Model file for the job. Use its own axes, mm. Face numbers are marked on the shaded views. A direction names the side the tool comes from. Round coordinates to 2 decimals unless told otherwise and drop trailing zeros. Order: outer loops, then holes, each group sorted by start corner. A loop starts at its lowest first (then second) coordinate and runs counter-clockwise, first axis right, second up. Notation, with made-up numbers: (85, 37) - (101, 37) arc R19 ccw to (101, 62) - close; hole circle Ø6 at (-17.5, 5.5). An arc over 180 degrees is marked (long way). Put each result on its own line as item: value. Start each with the question number.
Item 1: Probe probe 1 along Z at (x, y) = (2.5, -1.4); probe 2 along Y at (x, z) = (3.5, -4.5); probe 3 along Y at (x, z) = (6, -2.75). List the from-to ranges inside material, lowest first.
Item 2: Saw through at A-A on z = -4. List the corners of the cut face in (x, y).
Item 3: Saw through at D-D on z = -6. List the corners of the cut face in (x, y), plus the area to 3 significant figures.
Item 4: Which spindle directions (+Z, -Z, +X, -X, +Y, -Y) get a long thin tool onto all of the face, cutting with end or side? Do the marked faces 4, 5 and 6. Say none if no direction does.
Item 5: Pin check, flat tips, straight feed: pin 1 Ø3 at (x, z) = (3.5, -4.5) entering from -Y; pin 2 Ø1.5 at (y, z) = (2, -2) entering from +X; pin 3 Ø1 at (x, y) = (3, -1.5) entering from +Z. Stop position of each tip, or through.
Item 6: Mould opens along Z. For the marked faces 1, 2 and 3 say: pulls with the +Z half, pulls with the -Z half, needs draft (parallel to the pull), parting line crosses it, or undercut.
Item 7: Saw through at C-C on x = 5.25. List the corners of the cut face in (y, z), plus the area to 3 significant figures.
Item 8: Saw through at B-B on y = 1. List the corners of the cut face in (x, z).
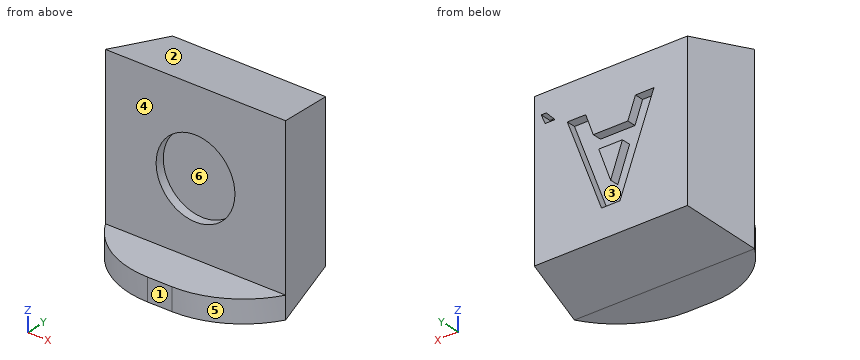
```python
from build123d import *

# Parameters (mm, degrees)
SKETCH1_W               = 8
SKETCH1_H               = 8
BOSS_EXTRUDE1_DEPTH     = 3
CUT_EXTRUDE1_DEPTH      = 12.704699911
CUT_EXTRUDE1_DEPTH_BACK = 12.704699911
CUT_EXTRUDE2_DEPTH      = 11
SKETCH4_R               = 1.75
CUT_EXTRUDE3_DEPTH      = 0.4
SKETCH5_W               = 8
SKETCH5_H               = 1
BOSS_EXTRUDE2_DEPTH     = 2
FILLET1_R               = 4
CUT_EXTRUDE4_DEPTH      = 0.4
CUT_EXTRUDE5_DEPTH      = 0.5


with BuildPart() as part:
    # Sketch1 → Boss-Extrude1 (new body)
    with BuildSketch(Plane(origin=(0, 0, 0), x_dir=(1, 0, 0), z_dir=(0, 1, 0))):
        with Locations((4, 4)):
            Rectangle(SKETCH1_W, SKETCH1_H)
    extrude(amount=BOSS_EXTRUDE1_DEPTH)

    # Sketch2 → Cut-Extrude1 (cut, two sides: drawn at the far end of the back side and taken through both)
    with BuildSketch(Plane.XY.offset(-CUT_EXTRUDE1_DEPTH_BACK)):
        Polygon((0, 0), (0.6, 3), (0, 3), align=None)
        Polygon((8, 0), (7.4, 3), (8, 3), align=None)
    extrude(amount=CUT_EXTRUDE1_DEPTH + CUT_EXTRUDE1_DEPTH_BACK, mode=Mode.SUBTRACT)

    # Sketch3 → Cut-Extrude2 (cut)
    with BuildSketch(Plane(origin=(0, 0, 0), x_dir=(0, 0, -1), z_dir=(1, 0, 0))):
        Polygon((0, 0), (0.6, 3), (0, 3), align=None)
        Polygon((8, 3), (7.4, 3), (8, 0), align=None)
    extrude(amount=CUT_EXTRUDE2_DEPTH, mode=Mode.SUBTRACT)

    # Sketch4 → Cut-Extrude3 (cut)
    with BuildSketch(Plane.XZ):
        with Locations(Location((4, -3.75, 0), (0, 0, 270))):
            Circle(SKETCH4_R)
    extrude(amount=-CUT_EXTRUDE3_DEPTH, mode=Mode.SUBTRACT)

    # Sketch5 → Boss-Extrude2 (add)
    with BuildSketch(Plane.XZ):
        with Locations((4, -7.5)):
            Rectangle(SKETCH5_W, SKETCH5_H)
    extrude(amount=BOSS_EXTRUDE2_DEPTH)

    # Fillet1
    # the kernel refuses this fillet: 4 mm, written as the material it takes off along each edge
    with BuildSketch(Plane(origin=(8, -2, -16.660254038), x_dir=(0, 1, 0), z_dir=(0, 0, 1)), Plane(origin=(0, -2, 1.660254038), x_dir=(0, 1, 0), z_dir=(0, 0, -1))) as fillet1_piece_1:
        with BuildLine():
            CenterArc((4, 3.464101615), FILLET1_R, 180, 60)
            Line((0, 3.464101615), (-0.08, 3.464101615))
            Line((-0.08, 3.464101615), (-0.08, 0))
            Line((-0.08, 0), (0, -0.08))
            ThreePointArc((0, -0.08), (1, -0.08), (1.96, -0.069282032))
            Line((1.96, -0.069282032), (2, 0))
        make_face()
    extrude(amount=18.320508076, mode=Mode.SUBTRACT)

    # Sketch6 → Cut-Extrude4 (cut)
    with BuildSketch(Plane(origin=(0, 3, 0), x_dir=(1, 0, 0), z_dir=(0, 1, 0))):
        Polygon((5.933857302, 2.141652068), (5.118152174, 2.141652068), (4.780812431, 3.064728992), (3.24555602, 3.064728992), (2.908216277, 2.141652068), (2.087703456, 2.141652068), (3.599722687, 6.141652068), (4.414626533, 6.141652068), align=None)
        Polygon((4.536421405, 3.731395658), (4.010780379, 5.167293094), (3.486741918, 3.731395658), align=None, mode=Mode.SUBTRACT)
    extrude(amount=-CUT_EXTRUDE4_DEPTH, mode=Mode.SUBTRACT)

    # Sketch7 → Cut-Extrude5 (cut)
    with BuildSketch(Plane(origin=(0, 3, 0), x_dir=(1, 0, 0), z_dir=(0, 1, 0))):
        Polygon((7.095591712, 1.44126633), (6.864822481, 1.44126633), (6.480207097, 1.85152274), (6.916104533, 1.85152274), align=None)
    extrude(amount=-CUT_EXTRUDE5_DEPTH, mode=Mode.SUBTRACT)


solid = part.part
```
Results found:
1. probe 1: z = -8 to -7
1. probe 2: y = 0.4 to 2.6
1. probe 3: y = 0 to 3
2. outline: (0, 0) - (2.27, 0) - (2.27, 0.4) - (5.73, 0.4) - (5.73, 0) - (8, 0) - (7.4, 3) - (5.23, 3) - (5.23, 2.6) - (4.44, 2.6) - (4.44, 3) - (3.58, 3) - (3.58, 2.6) - (2.79, 2.6) - (2.79, 3) - (0.6, 3) - close
3. outline: (0, 0) - (8, 0) - (7.4, 3) - (4.47, 3) - (4.47, 2.6) - (3.55, 2.6) - (3.55, 3) - (0.6, 3) - close
3. area: 21.8 mm²
4. face 4: +Z, +X, -X, -Y
4. face 5: +Z, -Z, +X, -Y
4. face 6: -Y
5. pin 1: stops at y = 0
5. pin 2: stops at x = 7.75
5. pin 3: stops at z = -7
6. face 1: needs draft
6. face 2: pulls with the +Z half
6. face 3: undercut
7. outline: (-1.94, -8) - (0, -8) - (3, -7.4) - (3, -3.94) - (2.6, -3.94) - (2.6, -2.14) - (3, -2.14) - (3, -0.6) - (0, 0) - (0, -2.53) - (0.4, -2.53) - (0.4, -4.97) - (0, -4.97) - (0, -7) - (-1.94, -7) - close
7. area: 22.4 mm²
8. outline: (0.2, -7.8) - (7.8, -7.8) - (7.8, -0.2) - (0.2, -0.2) - close
